Build history of the part. All positions in model axes, mm. Face numbers are marked on the shaded views. A direction names the side the tool comes from. Round coordinates to 2 decimals unless told otherwise and drop trailing zeros. Write each loop counter-clockwise with the first axis right and the second up, starting at its lowest first coordinate (ties: lowest second). Pieces come first, ordered by that corner, then holes. Notation, with made-up numbers: (84, -36) - (118, -36) arc R31 cw to (118, -8) - close; hole circle Ø4 at (46, -25.5). An arc over 180 degrees is marked (long way). Answer as a JSON object with one key per item and string values. Group by question number.
Item 1: Slice it at D-D, the plane z = -4.5. List the corners of the cut face in (x, y), then the cut area to 3 significant figures.
Item 2: Slice it at A-A, the plane x = -0.75. List the corners of the cut face in (y, z).
Item 3: Probe line 1 (Z direction, x = 2, y = -6.75); line 2 (Z direction, x = 1.25, y = -1.5); line 3 (X direction, y = -5.25, z = -4.75). List the from-to ranges inside material, lowest first. Write a range as from..to.
Item 4: Which spindle directions (+Z, -Z, +X, -X, +Y, -Y) get a long thin tool onto all of the face, cutting with end or side? Do the marked faces 5 and 6. Say none if no direction does.
Item 5: Slice it at C-C, the plane x = 2. List the corners of the cut face in (y, z), then the cut area to 3 significant figures.
Item 6: Two-plate mould, pull along Z, no slides. Class the marked faces 1, 2, 3 and 4: +Z half, -Z half, draft (parallel to the pull), parting line (faces both ways), or undercut.
Item 7: Slice it at B-B, the plane y = -0.25. List the corners of the cut face in (x, z), then the cut area to 3 significant figures.
Item 8: Flat gauge pins, fed straight in: pin 1 (4 mm diameter, centred on x = 1, z = 13, fed in from -Y); pin 2 (6.5 mm diameter, centred on x = 1.89, z = 3.27, fed in from +Y). Where does each tip first touch, or does it go through?
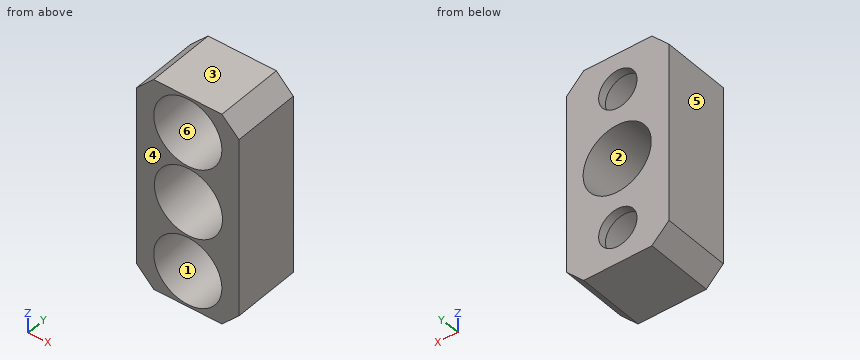
from build123d import *

# Parameters (mm, degrees)
F0_W     = 12
F0_H     = 25
F1_DEPTH = 8
F2_SIZE  = 2
F3_SIZE  = 2
F4_R     = 2.25
F5_DEPTH = 25
F6_R     = 4
F7_DEPTH = 7
F8_R     = 4
F9_DEPTH = 25


with BuildPart() as f1:
    # F0 (on Front) → F1 (new body)
    with BuildSketch(Plane.XZ):
        with Locations((1.81407, 3.270565)):
            Rectangle(F0_W, F0_H)
    extrude(amount=F1_DEPTH)

    # F2
    f2_edges = [f1.edges().sort_by_distance(p)[0] for p in [
        (-4.18593, -4, 15.770565),
    ]]
    chamfer(f2_edges, length=F2_SIZE)

    # F3
    f3_edges = [f1.edges().sort_by_distance(p)[0] for p in [
        (7.81407, -4, 15.770565),
        (7.81407, -4, -9.229435),
        (-4.18593, -4, -9.229435),
    ]]
    chamfer(f3_edges, length=F3_SIZE)

    # F4 (on face) → F5 (cut)
    with BuildSketch(Plane.XZ.offset(8)):
        with Locations((1.81407, -4.979435)):
            Circle(F4_R)
        with Locations((1.81407, 11.520565)):
            Circle(F4_R)
    extrude(amount=-F5_DEPTH, mode=Mode.SUBTRACT)

    # F6 (on face) → F7 (cut)
    with BuildSketch(Plane.XZ.offset(8)):
        with Locations((1.81407, 11.520565)):
            Circle(F6_R)
        with Locations((1.81407, -4.979435)):
            Circle(F6_R)
    extrude(amount=-F7_DEPTH, mode=Mode.SUBTRACT)

    # F8 (on Front) → F9 (cut)
    with BuildSketch(Plane.XZ):
        with Locations((1.887019, 3.270565)):
            Circle(F8_R)
    extrude(amount=F9_DEPTH, mode=Mode.SUBTRACT)


solid = f1.part
Geometry says:
{
 "1": {"outline": "(-4.19, -8) - (-2.16, -8) - (-2.16, -1) - (-0.38, -1) - (-0.38, 0) - (-4.19, 0) - close; (4.01, -1) - (5.79, -1) - (5.79, -8) - (7.81, -8) - (7.81, 0) - (4.01, 0) - close", "area": "36.0 mm^2"},
 "2": {"outline": "(-8, -9.23) - (0, -9.23) - (0, 0.26) - (-8, 0.26) - (-8, -1.91) - (-1, -1.91) - (-1, -8.05) - (-8, -8.05) - close; (-8, 6.28) - (0, 6.28) - (0, 15.77) - (-8, 15.77) - (-8, 14.59) - (-1, 14.59) - (-1, 8.45) - (-8, 8.45) - close"},
 "3": {"line 1": "z = -9.23..-8.98, -0.98..-0.73, 7.27..7.52, 15.52..15.77", "line 2": "z = -9.23..-8.94, -1.02..-0.68, 7.22..7.56, 15.48..15.77", "line 3": "x = -4.19..-2.18, 5.81..7.81"},
 "4": {"face 5": "+Z, -Z, -X, +Y, -Y", "face 6": "-Y"},
 "5": {"outline": "(-8, -9.23) - (0, -9.23) - (0, -7.22) - (-1, -7.22) - (-1, -8.98) - (-8, -8.98) - close; (-8, -0.98) - (-1, -0.98) - (-1, -2.74) - (0, -2.74) - (0, -0.73) - (-8, -0.73) - close; (-8, 7.27) - (0, 7.27) - (0, 9.28) - (-1, 9.28) - (-1, 7.52) - (-8, 7.52) - close; (-8, 15.52) - (-1, 15.52) - (-1, 13.76) - (0, 13.76) - (0, 15.77) - (-8, 15.77) - close", "area": "15.2 mm^2"},
 "6": {"face 1": "undercut", "face 2": "undercut", "face 3": "+Z half", "face 4": "draft"},
 "7": {"outline": "(-4.19, -7.23) - (-2.19, -9.23) - (5.81, -9.23) - (7.81, -7.23) - (7.81, 13.77) - (5.81, 15.77) - (-2.19, 15.77) - (-4.19, 13.77) - close; hole circle Ø8 at (1.89, 3.27); hole circle Ø4.5 at (1.81, -4.98); hole circle Ø4.5 at (1.81, 11.52)", "area": "210 mm^2"},
 "8": {"pin 1": "stops at y = -1", "pin 2": "passes through"}
}
